Check sheet for the modelled part. Datum: model origin and axes. Units: mm. Coordinates: 2 decimals unless noted, no trailing zeros. Write each loop counter-clockwise with the first axis right and the second up, starting at its lowest first coordinate (ties: lowest second). Pieces come first, ordered by that corner, then holes. Notation, with made-up numbers: (-18, 80.25) -> (39, 80.25) arc R24 cw to (39, 111.25) -> close; hole circle Ø3 at (51, -22.5). An arc over 180 degrees is marked (long way). One line per item, written item: value. Start each with the question number.
1) Scan lines: line 1 along Z through (x, y) = (2.4, 0); line 2 along Y through (x, z) = (0.35, -9); line 3 along Z through (x, y) = (4.25, -76). Record each from-to range of solid material in increasing order. Write a range as [from, to].
2) Sectioned sample at C-C on y = 0. Enter the section's corners in (x, z).
3) Sectioned sample at D-D on y = -112.5. Enter the section's corners in (x, z).
4) Sectioned sample at B-B on z = 0. Enter the section's corners in (x, y), plus the area to 3 significant figures.
5) Sectioned sample at A-A on x = 4.35. Give the number of separate pieces and of enclosed holes in the cut face, plus the area to 3 significant figures.
6) Gauge pin test, flat ends, axial feed: P1, Ø1.5, axis at x = 5.5, y = 118.5, coming from the +Z side; P2, Ø1.8, axis at x = 4, z = -2.5, coming from the +Y side; P3, Ø3, axis at x = 3.5, z = 27, coming from the -Y side. Record the tip position at first contact, or that the pin passes through.
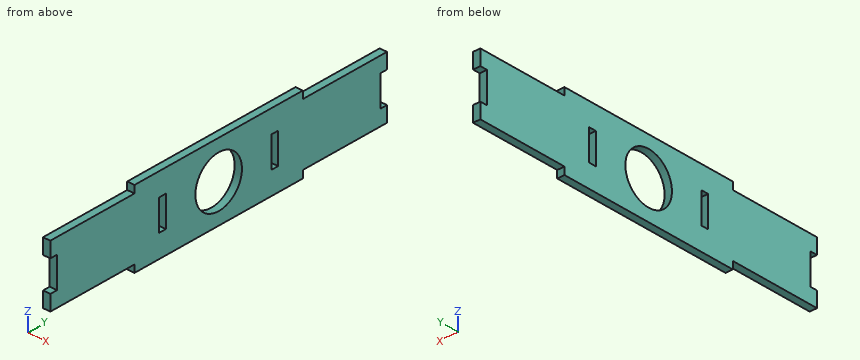
```python
from build123d import *

# Parameters (mm, degrees)
F0_W     = 150
F0_H     = 6
F1_DEPTH = 6
F2_R     = 20.75
F3_DEPTH = 6
F4_W     = 6
F4_H     = 25
F5_DEPTH = 6


with BuildPart() as f1:
    # F0 (on Right) → F1 (new body)
    with BuildSketch(Plane.YZ):
        Polygon((-75, 25), (-150, 25), (-150, 12.5), (-144, 12.5), (-144, -12.5), (-150, -12.5), (-150, -25), (-75, -25), (-75, -19), (75, -19), (75, -25), (150, -25), (150, -12.5), (144, -12.5), (144, 12.5), (150, 12.5), (150, 25), (75, 25), (75, 19), (-75, 19), align=None)
        with Locations((0, 28)):
            Rectangle(F0_W, F0_H)
        with Locations((0, 22)):
            Rectangle(F0_W, F0_H)
        with Locations((0, -28)):
            Rectangle(F0_W, F0_H)
        with Locations((0, -22)):
            Rectangle(F0_W, F0_H)
    extrude(amount=F1_DEPTH)

    # F2 (on face) → F3 (cut, through all)
    with BuildSketch(Plane.YZ.offset(6)):
        Circle(F2_R)
    extrude(amount=-F3_DEPTH, mode=Mode.SUBTRACT)

    # F4 (on face) → F5 (cut, through all)
    with BuildSketch(Plane.YZ.offset(6)):
        with Locations((-50, 0)):
            Rectangle(F4_W, F4_H)
        with Locations((50, 0)):
            Rectangle(F4_W, F4_H)
    extrude(amount=-F5_DEPTH, mode=Mode.SUBTRACT)


solid = f1.part
```
Answers:
1. line 1: z = [-31, -20.75], [20.75, 31]
1. line 2: y = [-144, -53], [-47, -18.7], [18.7, 47], [53, 144]
1. line 3: z = [-25, 25]
2. outline: (0, -31) -> (6, -31) -> (6, -20.75) -> (0, -20.75) -> close; (0, 20.75) -> (6, 20.75) -> (6, 31) -> (0, 31) -> close
3. outline: (0, -25) -> (6, -25) -> (6, 25) -> (0, 25) -> close
4. outline: (0, -144) -> (6, -144) -> (6, -53) -> (0, -53) -> close; (0, -47) -> (6, -47) -> (6, -20.75) -> (0, -20.75) -> close; (0, 20.75) -> (6, 20.75) -> (6, 47) -> (0, 47) -> close; (0, 53) -> (6, 53) -> (6, 144) -> (0, 144) -> close
4. area: 1,410 mm2
5. separate pieces: 1
5. enclosed holes: 3
5. area: 14,800 mm2
6. P1: stops at z = 25
6. P2: stops at y = 144
6. P3: stops at y = -75
